Autodesk Inventor part; units mm, degrees
ref_plane "YZ Plane" through (0, 0, 0) normal (1, 0, 0) x (0, 1, 0)
ref_plane "XZ Plane" through (0, 0, 0) normal (0, 1, 0) x (-1, 0, 0)
ref_plane "XY Plane" through (0, 0, 0) normal (0, 0, 1) x (1, 0, 0)
sketch "CD Nozzle Sketch" plane through (0, 0, 0) normal (1, 0, 0) x (0, 1, 0)
  line L0 (0, 0) -> (0, -80)
  line L1 (15.0042, -20) -> (15.0042, -1.5)
  line L2 (15.875, -1.5) -> (15.875, -20)
  arc A0 (6.35, -34.925) -> (15.875, -20) centre (-26.9286, -3.185) ccw
  line L3 (15.875, -1.5) -> (20.0042, -1.5)
  line L4 (20.0042, -1.5) -> (20.0042, 0)
  arc A1 (25.4, -79.375) -> (5, -35) centre (-81.1948, -101.502) ccw
  arc A2 (26.0708, -80) -> (6.35, -34.925) centre (-90.9256, -104.3355) ccw
  arc A3 (5, -35) -> (15.0042, -20) centre (-26.6763, -3.0373) ccw
  line L5 (16.5042, 0) -> (16.5042, -0.75)
  line L6 (16.5042, -0.75) -> (17.5042, -0.75)
  line L7 (17.5042, -0.75) -> (17.5042, 0)
  line L8 (17.5042, 0) -> (20.0042, 0)
  line L9 (0, 1) -> (0, 0)
  line L10 (0, 1) -> (0, 0)
  line L11 (0, 3.175) -> (0, 0)
  line L12 (0, -0.75) -> (0, 0)
  line L13 (0, 0) -> (0, -1.5)
  line L14 (15.0042, -1.5) -> (0, -1.5)
  line L15 (0, 0) -> (16.5042, 0)
  line L16 (26.0708, -80) -> (0, -80)
  line L17 (0, -79.375) -> (25.4, -79.375)
  dimension "d5" = 80
  dimension "d34" = 45
  dimension "d39" = 35
  dimension "d40" = 5
revolve "CD Nozzle" add sketch "CD Nozzle Sketch" angle 360 about axis through (0, 0, 0) along (0, 0, -1) contours L15 L5 L6 L7 L8 L4 L3 L2 A0 A2 L16 L0 L17 A1 A3 L1 L14
fillet "Fillet14" radius 15 1 edges at (0, -15.875, -20)
fillet "Fillet15" radius 10 1 edges at (0, -6.35, -34.925)
fillet "Fillet16" radius 10 1 edges at (0, -5, -35)
fillet "Fillet17" radius 10 1 edges at (0, -15.0042, -20)
properties part number "alpha-i-for-cfd" material "Steel, Mild"
Input: part model. Units: mm. Frame: model coordinates. A direction names the side the tool comes from. Coordinates: 2 decimals unless noted, no trailing zeros. Write each loop counter-clockwise with the first axis right and the second up, starting at its lowest first coordinate (ties: lowest second). Pieces come first, ordered by that corner, then holes. Notation, with made-up numbers: M -27,44 L 12,44 A32 ccw 12,70 Z; hole C 33,30.25 d2. An arc over 180 degrees is marked long. Answer as a JSON object with one key per item and string values. Group by question number.
(1) Section B-B on x = -19. Give the number of separate pieces and of enclosed holes in the cut face, plus the area to 3 significant figures.
(2) Section A-A on z = -14. Output: boundary loops of the cut face in (x, y) (3 decimals).
(3) Set-up query: faces 4 (the face through (5, -16, -0.75)), 5 (the face through (0, 0, 0)), 6 (the face through (0, 0, -79.375)). Return all of +Z, -Z, +X, -X, +Y, -Y with unobstructed straight access to the full face (end or side cutting, diameter ignored); none if empty.
(4) Contact query for flat-ended pins moving along their axis: P1, Ø2, axis at x = -10, z = -21, coming from the +Y side; P2, Ø8, axis at x = 9, z = -10.5, coming from the +Y side; P3, Ø1, axis at y = -3, z = -38, coming from the -X side. Output: stop coordinate, or through.
(5) Ray query, line 1 along X through (y, z) = (0, -0.5); line 2 along X through (y, z) = (0, -9) (3 decimals); line 3 along Z through (x, y) = (-14, 10) (3 decimals). Return the intervals inside material, ascending. Write a range as [from, to].
(6) Mould query, pull axis Y, two halves, no side actions, for faces 1 (the face through (-4.51, 14.31, -9.59)), 2 (the face through (-15.497, -3.441, -9.291)), 3 (the face through (0, 0, -80)). Classes: pulls with the +Y half, pulls with the -Y half, needs draft (parallel to the pull), parting line crosses it, or undercut.
Result set:
{
 "1": {"separate pieces": "2", "enclosed holes": "1", "area": "97.1 mm2"},
 "2": {"outline": "C 0,0 d31.75; hole C 0,0 d30.008"},
 "3": {"face 4": "+Z", "face 5": "+Z, +X, -X, +Y, -Y", "face 6": "none"},
 "4": {"P1": "stops at y = 12.44", "P2": "stops at y = 15.07", "P3": "stops at x = -8.8"},
 "5": {"line 1": "x = [-20, -17.5], [-16.5, 16.5], [17.5, 20]", "line 2": "x = [-15.875, -15.004], [15.004, 15.875]", "line 3": "z = [-80, -79.375], [-54.923, -53.461], [-1.5, -0.75]"},
 "6": {"face 1": "undercut", "face 2": "parting line crosses it", "face 3": "needs draft"}
}
